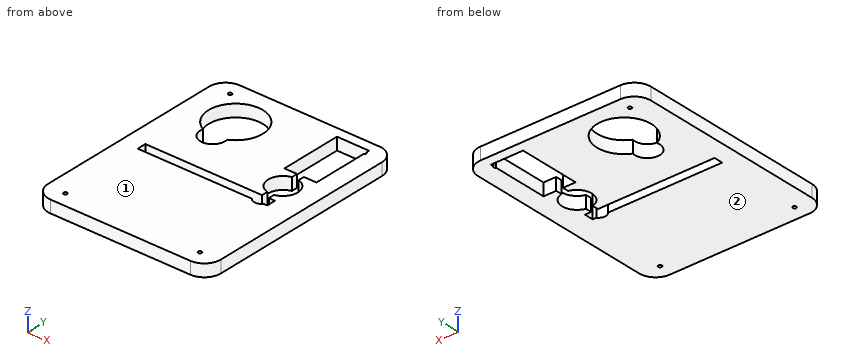
```python
from build123d import *

# Parameters (mm, degrees)
BOSS_EXTRUDE1_DEPTH         = 12.7
CUT_EXTRUDE1_DEPTH          = 13.7
F_27_0_144_DIAMETER_HOLE1_D = 3.6576


with BuildPart() as part:
    # Sketch1 → Boss-Extrude1 (new body)
    with BuildSketch(Plane(origin=(0, 0, 0), x_dir=(0, 1, 0), z_dir=(0, 0, 1))):
        with BuildLine():
            Line((-97.2566, -88.9), (97.2566, -88.9))
            ThreePointArc((97.2566, -88.9), (109.308103714, -83.908103714), (114.3, -71.8566))
            Line((114.3, -71.8566), (114.3, 71.8566))
            ThreePointArc((114.3, 71.8566), (109.308103714, 83.908103714), (97.2566, 88.9))
            Line((97.2566, 88.9), (-97.2566, 88.9))
            ThreePointArc((-97.2566, 88.9), (-109.308103714, 83.908103714), (-114.3, 71.8566))
            Line((-114.3, 71.8566), (-114.3, -71.8566))
            ThreePointArc((-114.3, -71.8566), (-109.308103714, -83.908103714), (-97.2566, -88.9))
        make_face()
    extrude(amount=BOSS_EXTRUDE1_DEPTH)

    # Sketch6 → Cut-Extrude1 (cut, through all)
    with BuildSketch(Plane.XY.offset(12.7)):
        with BuildLine():
            Line((49.8475, 4.691829089), (49.8475, -1.7145))
            Line((49.8475, -1.7145), (-70.1675, -1.7145))
            Line((-70.1675, -1.7145), (-70.1675, -10.9855))
            Line((-70.1675, -10.9855), (47.292145856, -10.9855))
            ThreePointArc((47.292145856, -10.9855), (53.34, -13.97), (59.387854144, -10.9855))
            Line((59.387854144, -10.9855), (63.1825, -10.9855))
            Line((63.1825, -10.9855), (63.1825, -1.7145))
            Line((63.1825, -1.7145), (56.8325, -1.7145))
            Line((56.8325, -1.7145), (56.8325, 4.691829089))
            ThreePointArc((56.8325, 4.691829089), (68.58, 19.52625), (56.8325, 34.360670911))
            Line((56.8325, 34.360670911), (56.8325, 40.64))
            Line((56.8325, 40.64), (69.85, 40.64))
            Line((69.85, 40.64), (69.85, 104.14))
            Line((69.85, 104.14), (36.83, 104.14))
            Line((36.83, 104.14), (36.83, 40.64))
            Line((36.83, 40.64), (49.8475, 40.64))
            Line((49.8475, 40.64), (49.8475, 34.360670911))
            ThreePointArc((49.8475, 34.360670911), (38.1, 19.52625), (49.8475, 4.691829089))
        make_face()
        with BuildLine():
            ThreePointArc((-25.732344403, 44.796363636), (-38.1, 97.79), (-50.467655597, 44.796363636))
            ThreePointArc((-50.467655597, 44.796363636), (-38.1, 29.21), (-25.732344403, 44.796363636))
        make_face()
    extrude(amount=-CUT_EXTRUDE1_DEPTH, mode=Mode.SUBTRACT)

    # #27 (0.144) Diameter Hole1 (through all)
    with Locations(Plane.XY.offset(12.7)):
        with Locations((-69.21913, 99.508615), (-69.21913, -99.508615), (69.21913, -99.508615), (69.21913, 99.508615)):
            Hole(F_27_0_144_DIAMETER_HOLE1_D / 2)


solid = part.part
```
Design review of the part built by this model. Coordinates are the model's own, in mm. Face numbers are marked on the shaded views. Coordinates: 2 decimals unless noted, no trailing zeros. Order: outer loops, then holes, each group sorted by start corner. A loop starts at its lowest first (then second) coordinate and runs counter-clockwise, first axis right, second up. Notation, with made-up numbers: (57.5, -22.75) - (110.5, -22.75) arc R17 ccw to (110.5, 8.25) - close; hole circle Ø9 at (-30, 66). An arc over 180 degrees is marked (long way). Answer in a Markdown table with one row per item.
(1) Wall thickness on line 1 along X through (y, z) = (69.85, 5); line 2 along X through (y, z) = (41.91, 9.5); line 3 along X through (y, z) = (0, 3.75): over which ranges is each line inside the solid? List them lowest first. Write a range as from..to.
Checked values:
| item | result |
|---|---|
| line 1 | -88.9..-66.04, -10.16..36.83, 69.85..88.9 |
| line 2 | -88.9..-50.8, -25.4..36.83, 69.85..88.9 |
| line 3 | -88.9..49.85, 56.83..88.9 |
(2) Consider section C-C on x = -1. State the section outline as (y, z) points.
Checked values:
| item | result |
|---|---|
| outline | (-114.3, 0) - (-10.99, 0) - (-10.99, 12.7) - (-114.3, 12.7) - close; (-1.71, 0) - (114.3, 0) - (114.3, 12.7) - (-1.71, 12.7) - close |
(3) Consider section B-B on y = 69.85. State the section outline as (x, z) points.
Checked values:
| item | result |
|---|---|
| outline | (-88.9, 0) - (-66.04, 0) - (-66.04, 12.7) - (-88.9, 12.7) - close; (-10.16, 0) - (36.83, 0) - (36.83, 12.7) - (-10.16, 12.7) - close; (69.85, 0) - (88.9, 0) - (88.9, 12.7) - (69.85, 12.7) - close |
(4) Consider section D-D on y = -6. State the section outline as (x, z) points, plus the area to 3 significant figures.
Checked values:
| item | result |
|---|---|
| outline | (-88.9, 0) - (-70.17, 0) - (-70.17, 12.7) - (-88.9, 12.7) - close; (63.18, 0) - (88.9, 0) - (88.9, 12.7) - (63.18, 12.7) - close |
| area | 565 mm^2 |
(5) The part is to be moulded in two halves that separate along Z. For the marked faces 1 and 2, say which applies: released by +Z, released by -Z, zero draft, split by the parting line, or undercut.
Checked values:
| item | result |
|---|---|
| face 1 | released by +Z |
| face 2 | released by -Z |
(6) Consider section A-A on x = -38.1. State the section outline as (y, z) points.
Checked values:
| item | result |
|---|---|
| outline | (-114.3, 0) - (-10.99, 0) - (-10.99, 12.7) - (-114.3, 12.7) - close; (-1.71, 0) - (29.21, 0) - (29.21, 12.7) - (-1.71, 12.7) - close; (97.79, 0) - (114.3, 0) - (114.3, 12.7) - (97.79, 12.7) - close |
(7) Clearance check with flat-ended pins moving along their axes: pin 1 (6 mm diameter, centred on x = 69.22, y = -99.51, fed in from -Z); pin 2 (1.5 mm diameter, centred on y = 103, z = 5.5, fed in from -X). State where each tip first meets the part, or that it passes through.
Checked values:
| item | result |
|---|---|
| pin 1 | z = 0 |
| pin 2 | x = -88.15 |
